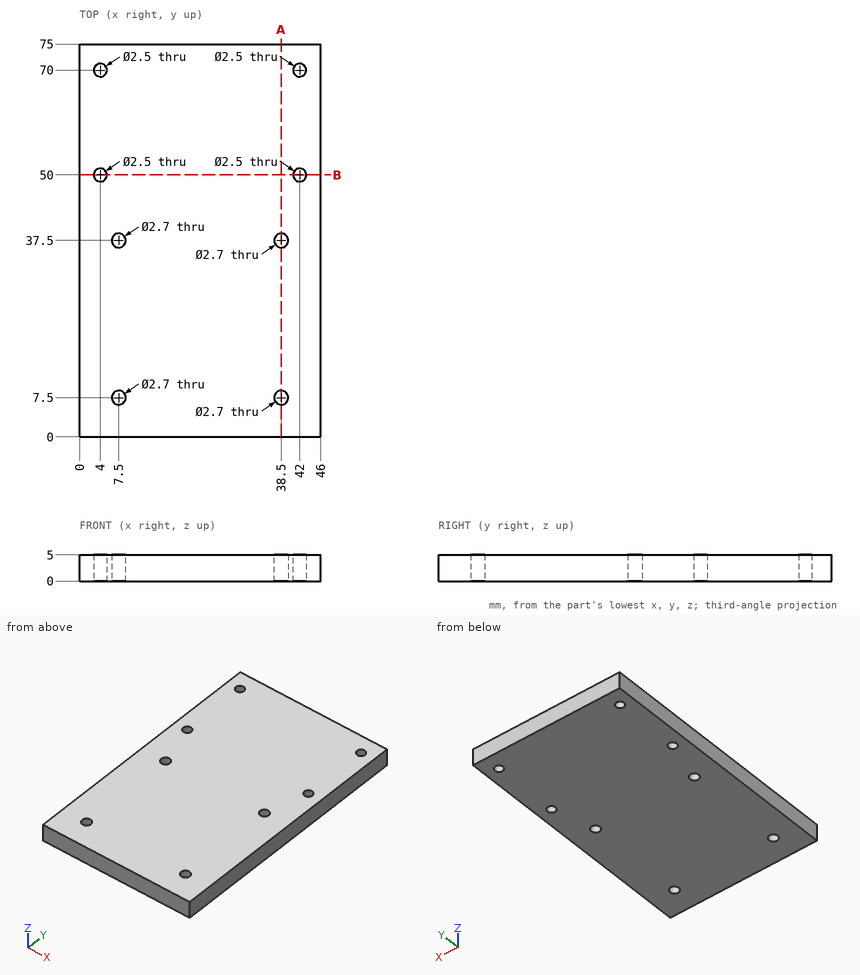
The figure shows three views and two pictorial views of one solid part (mm, origin at its lowest corner). Answer the questions. Round coordinates to 2 decimals unless told otherwise and drop trailing zeros. Write each loop counter-clockwise with the first axis right and the second up, starting at its lowest first coordinate (ties: lowest second). Pieces come first, ordered by that corner, then holes. Notation, with made-up numbers: (1.25, 6) - (54.25, 6) arc R10 ccw to (54.25, 22) - close; hole circle Ø1 at (30.5, -39). An arc over 180 degrees is marked (long way). Answer in a Markdown table with one row per item. Add a question column.
1. A cutting plane is placed at A-A, the plane x = 38.5. Determine the outline of the cut face in (y, z).
2. A cutting plane is placed at B-B, the plane y = 50. Determine the outline of the cut face in (x, z).
3. Find the intervals of material crossed by line 1 along Y through (x, z) = (4, 3.1); line 2 along Y through (x, z) = (7.5, 2.25); line 3 along X through (y, z) = (70, 4), in increasing order. Write a range as from..to.
Worked out:
| question | item | result |
|---|---|---|
| 1 | outline | (0, 0) - (6.15, 0) - (6.15, 5) - (0, 5) - close; (8.85, 0) - (36.15, 0) - (36.15, 5) - (8.85, 5) - close; (38.85, 0) - (75, 0) - (75, 5) - (38.85, 5) - close |
| 2 | outline | (0, 0) - (2.75, 0) - (2.75, 5) - (0, 5) - close; (5.25, 0) - (40.75, 0) - (40.75, 5) - (5.25, 5) - close; (43.25, 0) - (46, 0) - (46, 5) - (43.25, 5) - close |
| 3 | line 1 | 0..48.75, 51.25..68.75, 71.25..75 |
| 3 | line 2 | 0..6.15, 8.85..36.15, 38.85..75 |
| 3 | line 3 | 0..2.75, 5.25..40.75, 43.25..46 |
